from build123d import *

# Parameters (mm, degrees)
SKETCH1_R           = 18.5
BOSS_EXTRUDE1_DEPTH = 3
BOSS_EXTRUDE2_START = -3
BOSS_EXTRUDE2_DEPTH = 3
SKETCH3_R           = 1.6
CUT_EXTRUDE1_DEPTH  = 3


with BuildPart() as part:
    # Sketch1 → Boss-Extrude1 (new body)
    with BuildSketch(Plane.XY):
        Circle(SKETCH1_R)
    extrude(amount=BOSS_EXTRUDE1_DEPTH)

    # Sketch2 → Boss-Extrude2 (add)
    with BuildSketch(Plane.XY.offset(3).offset(BOSS_EXTRUDE2_START)):
        with BuildLine():
            Line((0.845055361, 22.340372437), (0, 18.5))
            ThreePointArc((0, 18.5), (3.741363138, 18.117731698), (7.32810957, 16.986724526))
            Line((7.32810957, 16.986724526), (8.152336268, 20.732440653))
            ThreePointArc((8.152336268, 20.732440653), (8.018246407, 21.485969914), (7.390604906, 21.923979714))
            Line((7.390604906, 21.923979714), (2.036594422, 23.102103799))
            ThreePointArc((2.036594422, 23.102103799), (1.283065161, 22.968013938), (0.845055361, 22.340372437))
        make_face()
        with BuildLine():
            Line((14.839691312, 11.046880182), (17.426350635, 13.878652154))
            ThreePointArc((17.426350635, 13.878652154), (17.686990039, 14.598272567), (17.362441455, 15.291420931))
            Line((17.362441455, 15.291420931), (13.314794406, 18.98871156))
            ThreePointArc((13.314794406, 18.98871156), (12.595173993, 19.249350964), (11.902025629, 18.92480238))
            Line((11.902025629, 18.92480238), (9.25, 16.02146997))
            ThreePointArc((9.25, 16.02146997), (12.298981371, 13.81973434), (14.839691312, 11.046880182))
        make_face()
        with BuildLine():
            Line((18.374989752, 2.147033214), (22.030988422, 3.306090019))
            ThreePointArc((22.030988422, 3.306090019), (22.616518974, 3.798979875), (22.682025838, 4.561538259))
            Line((22.682025838, 4.561538259), (21.025305982, 9.787309393))
            ThreePointArc((21.025305982, 9.787309393), (20.532416125, 10.372839945), (19.769857741, 10.438346808))
            Line((19.769857741, 10.438346808), (16.02146997, 9.25))
            ThreePointArc((16.02146997, 9.25), (17.561097478, 5.818750327), (18.374989752, 2.147033214))
        make_face()
        with BuildLine():
            Line((16.986724526, -7.32810957), (20.732440653, -8.152336268))
            ThreePointArc((20.732440653, -8.152336268), (21.485969914, -8.018246407), (21.923979714, -7.390604906))
            Line((21.923979714, -7.390604906), (23.102103799, -2.036594422))
            ThreePointArc((23.102103799, -2.036594422), (22.968013938, -1.283065161), (22.340372437, -0.845055361))
            Line((22.340372437, -0.845055361), (18.5, 0))
            ThreePointArc((18.5, 0), (18.117731698, -3.741363138), (16.986724526, -7.32810957))
        make_face()
        with BuildLine():
            Line((11.046880182, -14.839691312), (13.878652154, -17.426350635))
            ThreePointArc((13.878652154, -17.426350635), (14.598272567, -17.686990039), (15.291420931, -17.362441455))
            Line((15.291420931, -17.362441455), (18.98871156, -13.314794406))
            ThreePointArc((18.98871156, -13.314794406), (19.249350964, -12.595173993), (18.92480238, -11.902025629))
            Line((18.92480238, -11.902025629), (16.02146997, -9.25))
            ThreePointArc((16.02146997, -9.25), (13.81973434, -12.298981371), (11.046880182, -14.839691312))
        make_face()
        with BuildLine():
            Line((3.222223056, -21.766447889), (3.306090019, -22.030988422))
            ThreePointArc((3.306090019, -22.030988422), (3.798979875, -22.616518974), (4.561538259, -22.682025838))
            Line((4.561538259, -22.682025838), (9.787309393, -21.025305982))
            ThreePointArc((9.787309393, -21.025305982), (10.372839945, -20.532416125), (10.438346808, -19.769857741))
            Line((10.438346808, -19.769857741), (10.329178092, -19.425508197))
            Line((10.329178092, -19.425508197), (9.25, -16.02146997))
            ThreePointArc((9.25, -16.02146997), (5.818750327, -17.561097478), (2.147033214, -18.374989752))
            Line((2.147033214, -18.374989752), (3.222223056, -21.766447889))
        make_face()
        with BuildLine():
            Line((-7.32810957, -16.986724526), (-8.152336268, -20.732440653))
            ThreePointArc((-8.152336268, -20.732440653), (-8.018246407, -21.485969914), (-7.390604906, -21.923979714))
            Line((-7.390604906, -21.923979714), (-2.036594422, -23.102103799))
            ThreePointArc((-2.036594422, -23.102103799), (-1.283065161, -22.968013938), (-0.845055361, -22.340372437))
            Line((-0.845055361, -22.340372437), (0, -18.5))
            ThreePointArc((0, -18.5), (-3.741363138, -18.117731698), (-7.32810957, -16.986724526))
        make_face()
        with BuildLine():
            Line((-14.839691312, -11.046880182), (-17.426350635, -13.878652154))
            ThreePointArc((-17.426350635, -13.878652154), (-17.686990039, -14.598272567), (-17.362441455, -15.291420931))
            Line((-17.362441455, -15.291420931), (-13.314794406, -18.98871156))
            ThreePointArc((-13.314794406, -18.98871156), (-12.595173993, -19.249350964), (-11.902025629, -18.92480238))
            Line((-11.902025629, -18.92480238), (-9.25, -16.02146997))
            ThreePointArc((-9.25, -16.02146997), (-12.298981371, -13.81973434), (-14.839691312, -11.046880182))
        make_face()
        with BuildLine():
            Line((-18.374989752, -2.147033214), (-22.030988422, -3.306090019))
            ThreePointArc((-22.030988422, -3.306090019), (-22.616518974, -3.798979875), (-22.682025838, -4.561538259))
            Line((-22.682025838, -4.561538259), (-21.025305982, -9.787309393))
            ThreePointArc((-21.025305982, -9.787309393), (-20.532416125, -10.372839945), (-19.769857741, -10.438346808))
            Line((-19.769857741, -10.438346808), (-16.02146997, -9.25))
            ThreePointArc((-16.02146997, -9.25), (-17.561097478, -5.818750327), (-18.374989752, -2.147033214))
        make_face()
        with BuildLine():
            Line((-16.986724526, 7.32810957), (-20.732440653, 8.152336268))
            ThreePointArc((-20.732440653, 8.152336268), (-21.485969914, 8.018246407), (-21.923979714, 7.390604906))
            Line((-21.923979714, 7.390604906), (-23.102103799, 2.036594422))
            ThreePointArc((-23.102103799, 2.036594422), (-22.968013938, 1.283065161), (-22.340372437, 0.845055361))
            Line((-22.340372437, 0.845055361), (-18.5, 0))
            ThreePointArc((-18.5, 0), (-18.117731698, 3.741363138), (-16.986724526, 7.32810957))
        make_face()
        with BuildLine():
            Line((-11.046880182, 14.839691312), (-13.878652154, 17.426350635))
            ThreePointArc((-13.878652154, 17.426350635), (-14.598272567, 17.686990039), (-15.291420931, 17.362441455))
            Line((-15.291420931, 17.362441455), (-18.98871156, 13.314794406))
            ThreePointArc((-18.98871156, 13.314794406), (-19.249350964, 12.595173993), (-18.92480238, 11.902025629))
            Line((-18.92480238, 11.902025629), (-16.02146997, 9.25))
            ThreePointArc((-16.02146997, 9.25), (-13.81973434, 12.298981371), (-11.046880182, 14.839691312))
        make_face()
        with BuildLine():
            Line((-2.147033214, 18.374989752), (-3.306090019, 22.030988422))
            ThreePointArc((-3.306090019, 22.030988422), (-3.798979875, 22.616518974), (-4.561538259, 22.682025838))
            Line((-4.561538259, 22.682025838), (-9.787309393, 21.025305982))
            ThreePointArc((-9.787309393, 21.025305982), (-10.372839945, 20.532416125), (-10.438346808, 19.769857741))
            Line((-10.438346808, 19.769857741), (-9.25, 16.02146997))
            ThreePointArc((-9.25, 16.02146997), (-5.818750327, 17.561097478), (-2.147033214, 18.374989752))
        make_face()
    extrude(amount=BOSS_EXTRUDE2_DEPTH)

    # Sketch3 → Cut-Extrude1 (cut)
    with BuildSketch(Plane.XY.offset(3)):
        Circle(SKETCH3_R)
    extrude(amount=-CUT_EXTRUDE1_DEPTH, mode=Mode.SUBTRACT)


solid = part.part
Read the model definition and answer for the solid it produces. Units are mm, in the model's axes. A direction names the side the tool comes from. Give positions to 0.01 mm unless a question says otherwise; leave off trailing zeros. Answer as a JSON object with one key per item and string values. Group by question number.
1) Each of these flat-tipped pins is pushed along its axis until it touches: P1, Ø1.9, axis at x = 0, y = 0, coming from the +Z side; P2, Ø1, axis at x = -10.5, z = 1.5, coming from the +Y side. Where does it stop, or does it pass through?
2) The mould has two halves that part along Y. Classify faces 4 (the flat face through (4.751, 22.505, 1.479)), 5 (the cylindrical face through (18.47, 1.06, 1.48)), 6 (the cylindrical face through (1.06, -18.47, 1.48)): +Y half, -Y half, draft (parallel to the pull), parting line (faces both ways), or undercut.
3) Consider L1, parallel to X at y = -17.5, z = 1.25; L2, parallel to Y at x = 17, z = 2.55; L3, parallel to X at y = 1, z = 1.5. Determine where each line is inside the solid, lowest interval first. Write a range as from..to.
4) A tool of negligible diameter and unlimited length cuts with its end or side. For faces 1 (the cylindrical face through (16.525, -8.317, 1.479)), 2 (the flat face through (-20.18, -2.72, 1.48)), 3 (the flat face through (16.11, 12.44, 1.48)), from which of +Z, -Z, +X, -X, +Y, -Y can it reach the whole face along a straight path? Write none if from no direction.
Values follow:
{
 "1": {"P1": "passes through", "P2": "stops at y = 20.93"},
 "2": {"face 4": "+Y half", "face 5": "undercut", "face 6": "-Y half"},
 "3": {"L1": "x = -14.94..-10.6, -7.44..9.72, 13.97..15.14", "L2": "y = -15.49..-10.14, -7.33..9.56, 13.41..15.62", "L3": "x = -22.7..-1.25, 1.25..18.47"},
 "4": {"face 1": "+Z, -Z", "face 2": "+Z, -Z, -X", "face 3": "+Z, -Z, +X"}
}
